Answer from the drawing. Dimensions are ordinates in mm from the lowest x, y and z of the part. Give positions to 0.01 mm unless a question says otherwise; leave off trailing zeros. Order: outer loops, then holes, each group sorted by start corner. A loop starts at its lowest first (then second) coordinate and runs counter-clockwise, first axis right, second up. Notation, with made-up numbers: (5, -9.75) -> (21, -9.75) arc R24 cw to (21, 29.25) -> close; hole circle Ø1 at (24, 49.5). An arc over 180 degrees is marked (long way). Write item = value, one per line. Start each with the question number.
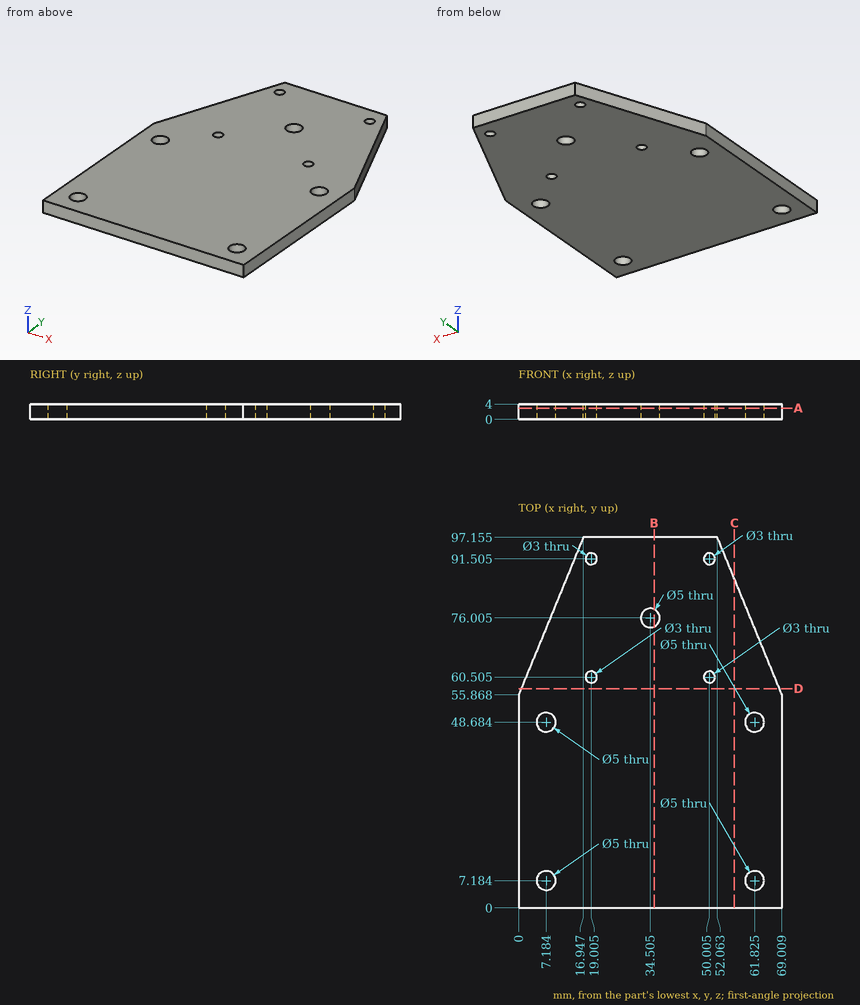
Item 1: A cutting plane is placed at D-D, the plane y = 57.5. Write down the section's boundary in (x, z), plus the area to 3 significant figures.
Item 2: A flat-ended cylindrical pin translates along its axis: pin 1 (1 mm diameter, centred on x = 23, z = 1, fed in from -Y). Find the tip coordinate at first contact, or state that the pin passes through.
Item 3: A cutting plane is placed at B-B, the plane x = 35.5. Write down the section's boundary in (y, z) (1 decimal).
Item 4: A cutting plane is placed at C-C, the plane x = 56.5. Write down the section's boundary in (y, z) (1 decimal).
Item 5: Consider L1, parallel to Y at x = 62, z = 0.2 (1 decimal); L2, parallel to Y at x = 35, z = 1.4 (1 decimal); L3, parallel to X at y = 8.5, z = 1.8. Determine where each line is inside the solid, lowest interval first. Write a range as from..to.
Item 6: A cutting plane is placed at A-A, the plane z = 2.9. Count the separate pieces of the cut face and the enclosed holes in it, plus the area to 3 significant figures.
Check values:
q1.outline = (0.67, 0) -> (68.34, 0) -> (68.34, 4) -> (0.67, 4) -> close
q1.area = 271 mm^2
q2.pin_1 = 0
q3.outline = (0, 0) -> (73.7, 0) -> (73.7, 4) -> (0, 4) -> close; (78.3, 0) -> (97.2, 0) -> (97.2, 4) -> (78.3, 4) -> close
q4.outline = (0, 0) -> (86.3, 0) -> (86.3, 4) -> (0, 4) -> close
q5.L1 = 0..4.7, 9.7..46.2, 51.2..72.9
q5.L2 = 0..73.6, 78.5..97.2
q5.L3 = 0..5.06, 9.31..59.7, 63.95..69.01
q6.separate_pieces = 1
q6.enclosed_holes = 9
q6.area = 5,880 mm^2
